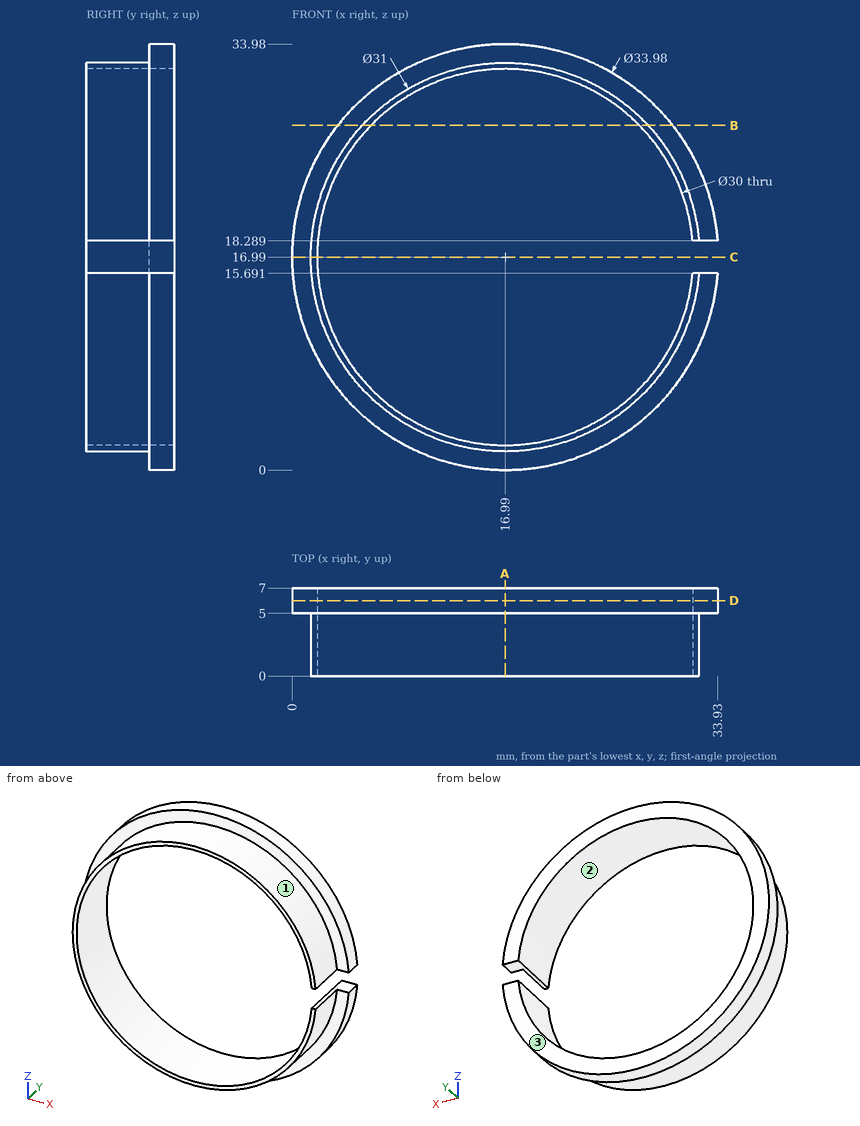
Design review of the part shown in the three views and the two pictorial views. Dimensions are in mm from the part's minimum x, y and z. Coordinates: 2 decimals unless noted, no trailing zeros. Loops run counter-clockwise (first coordinate to the right, second up) from the corner with the lowest first, then second, coordinate; pieces in that order, holes last.
Q1. The part is to be moulded in two halves that separate along X. For the marked faces 1, 2 and 3, say which applies: +X half, -X half, draft (parallel to the pull), parting line (faces both ways), or undercut.
Reported:
face 1: parting line
face 2: undercut
face 3: draft
Q2. We need section D-D on y = 6. State the section outline as (x, z) points.
Reported:
outline: (31.93, 15.69) arc R15 cw (long way) to (31.93, 18.29) - (33.93, 18.29) arc R16.99 ccw (long way) to (33.93, 15.69) - close
Q3. We need section A-A on x = 16.99. State the section outline as (y, z) points.
Reported:
outline: (0, 1.49) - (5, 1.49) - (5, 0) - (7, 0) - (7, 1.99) - (0, 1.99) - close; (0, 31.99) - (7, 31.99) - (7, 33.98) - (5, 33.98) - (5, 32.49) - (0, 32.49) - close
Q4. We need section B-B on z = 27.5. State the section outline as (x, y) points.
Reported:
outline: (3.64, 5) - (5.6, 5) - (5.6, 0) - (6.29, 0) - (6.29, 7) - (3.64, 7) - close; (27.69, 0) - (28.38, 0) - (28.38, 5) - (30.34, 5) - (30.34, 7) - (27.69, 7) - close
Q5. We need section C-C on z = 16.99. State the section outline as (x, y) points.
Reported:
outline: (0, 5) - (1.49, 5) - (1.49, 0) - (1.99, 0) - (1.99, 7) - (0, 7) - close
Q6. For pin 1 (2 mm diameter, centred on y = 1.5, z = 28, fed in from +X) (1 decimal); pin 2 (0.6 mm diameter, centred on x = 33, y = 3.5, fed in from -Z); pin 3 (1.5 mm diameter, centred on y = 5.5, z = 8, fed in from +X); pin 4 (3 mm diameter, centred on y = 2, z = 26.5, fed in from +X), all flat-tipped, find the tip position at first contact; note any pin that passes through.
Reported:
pin 1: stops at x = 28.8
pin 2: passes through
pin 3: stops at x = 31.85
pin 4: stops at x = 30.26
Q7. To check wall thickness, follow line 1 (Z direction, x = 16.99, y = 5.5); line 2 (Z direction, x = 16.99, y = 3); line 3 (X direction, y = 3.25, z = 16.99). State the ranges of each line that lie inside material, in increasing order.
Reported:
line 1: z = 0 to 1.99, 31.99 to 33.98
line 2: z = 1.49 to 1.99, 31.99 to 32.49
line 3: x = 1.49 to 1.99
